Build history of the part. All positions in model axes, mm. A direction names the side the tool comes from. Round coordinates to 2 decimals unless told otherwise and drop trailing zeros. Write each loop counter-clockwise with the first axis right and the second up, starting at its lowest first coordinate (ties: lowest second). Pieces come first, ordered by that corner, then holes. Notation, with made-up numbers: (3.25, 27.25) - (30.25, 27.25) arc R23 ccw to (30.25, 55.25) - close; hole circle Ø5 at (-7, 50.25). An arc over 180 degrees is marked (long way). Answer as a JSON object with one key per item and string values. Group by question number.
Item 1: Slice it at B-B, the plane y = -42.5. List the corners of the cut face in (x, z).
Item 2: Two-plate mould, pull along X, no slides. Class faces 5 (the flat face through (60, -56, 20)), 6 (the flat face through (29.6, -54.2, 0)), 7 (the flat face through (50, -56, 15)), 8 (the flat face through (40, -100, 15)): +X half, -X half, draft (parallel to the pull), parting line (faces both ways), or undercut.
Item 3: Slice it at D-D, the plane y = -23.5. List the corners of the cut face in (x, z), then the cut area to 3 significant figures.
Item 4: Flat gauge pins, fed straight in: pin 1 (5 mm diameter, centred on x = 25.5, y = -26, fed in from -Z); pin 2 (10 mm diameter, centred on x = 14.5, z = 29.5, fed in from -Y); pin 3 (8 mm diameter, centred on y = -88, z = 28, fed in from -X). Where does each tip first touch, or does it go through?
Item 5: Which spindle directions (+Z, -Z, +X, -X, +Y, -Y) get a long thin tool onto all of the face, cutting with end or side? Do faces 1 (the flat face through (36, -54, 40)), 2 (the flat face through (15, -37.5, 15)), 3 (the flat face through (10, -50, 20)), 4 (the flat face through (30, -69, 15)). Say none if no direction does.
Item 6: Probe line 1 (Y direction, x = 19.5, z = 21.5); line 2 (Y direction, x = 36, z = 23); line 3 (X direction, y = -64, z = 24). List the from-to ranges inside material, lowest first. Write a range as from..to.
Item 7: Slice it at C-C, the plane z = 20.5. List the corners of the cut face in (x, y), then the cut area to 3 significant figures.
Item 8: Slice it at A-A, the plane x = 16.5. List the corners of the cut face in (y, z).
from build123d import *

# Parameters (mm, degrees)
SKETCH_1_W          = 60
SKETCH_1_H          = 50
SKETCH_1_W_2        = 40
SKETCH_1_H_2        = 60
EXTRUDE_1_DEPTH     = 40
SKETCH_3_W          = 20
SKETCH_3_H          = 62.5
CUT_EXTRUDE_1_DEPTH = 30


with BuildPart() as part:
    # 스케치1 → 보스-돌출1 (new body)
    with BuildSketch(Plane.XY):
        with Locations((30, -25)):
            Rectangle(SKETCH_1_W, SKETCH_1_H)
        with Locations((40, -80)):
            Rectangle(SKETCH_1_W_2, SKETCH_1_H_2)
    extrude(amount=EXTRUDE_1_DEPTH)

    # 스케치3 → 컷-돌출1 (cut)
    with BuildSketch(Plane(origin=(0, 0, 0), x_dir=(-1, 0, 0), z_dir=(0, 0, -1))):
        Polygon((0, -37.5), (0, -12.5), (-50, -12.5), (-50, -37.5), (-30, -37.5), align=None)
        with Locations((-40, -68.75)):
            Rectangle(SKETCH_3_W, SKETCH_3_H)
    extrude(amount=-CUT_EXTRUDE_1_DEPTH, mode=Mode.SUBTRACT)


solid = part.part
Geometry says:
{
 "1": {"outline": "(0, 0) - (30, 0) - (30, 30) - (50, 30) - (50, 0) - (60, 0) - (60, 40) - (0, 40) - close"},
 "2": {"face 5": "+X half", "face 6": "draft", "face 7": "undercut", "face 8": "undercut"},
 "3": {"outline": "(0, 30) - (50, 30) - (50, 0) - (60, 0) - (60, 40) - (0, 40) - close", "area": "900 mm^2"},
 "4": {"pin 1": "stops at z = 30", "pin 2": "stops at y = -50", "pin 3": "stops at x = 20"},
 "5": {"face 1": "+Z, +X, -X, +Y, -Y", "face 2": "-Z, -X", "face 3": "+Z, -Z, -X, -Y", "face 4": "-Z"},
 "6": {"line 1": "y = -50..-37.5, -12.5..0", "line 2": "y = -110..-100, -12.5..0", "line 3": "x = 20..30, 50..60"},
 "7": {"outline": "(0, -50) - (20, -50) - (20, -110) - (60, -110) - (60, 0) - (0, 0) - (0, -12.5) - (50, -12.5) - (50, -100) - (30, -100) - (30, -37.5) - (0, -37.5) - close", "area": "2,900 mm^2"},
 "8": {"outline": "(-50, 0) - (-37.5, 0) - (-37.5, 30) - (-12.5, 30) - (-12.5, 0) - (0, 0) - (0, 40) - (-50, 40) - close"}
}
